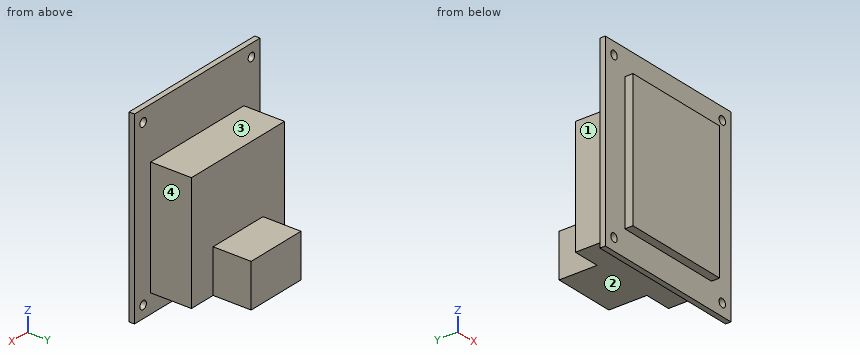
from build123d import *

# Parameters (mm, degrees)
SKETCH_1_W                  = 58
SKETCH_1_H                  = 69
EXTRUDE_351_DEPTH           = 2
SKETCH_2_W                  = 43
SKETCH_2_H                  = 43
EXTRUDE_607_DEPTH           = 15
SKETCH_3_W                  = 23
SKETCH_3_H                  = 16
EXTRUDE_850_DEPTH           = 14
SKETCH_4_W                  = 40
SKETCH_4_H                  = 50
EXTRUDE_1071_DEPTH          = 3
CUT_EXTRUDE_1381_DEPTH      = 54.593376456
CUT_EXTRUDE_1381_DEPTH_BACK = 54.593376456
SKETCH_7_R                  = 1.5


with BuildPart() as part:
    # Эскиз1 → Extrude 351 (new body)
    with BuildSketch(Plane.XZ):
        Rectangle(SKETCH_1_W, SKETCH_1_H)
    extrude(amount=-EXTRUDE_351_DEPTH)

    # Эскиз2 → Extrude 607 (add)
    with BuildSketch(Plane(origin=(0, 2, 0), x_dir=(-1, 0, 0), z_dir=(0, 1, 0))):
        with Locations((0, -6)):
            Rectangle(SKETCH_2_W, SKETCH_2_H)
    extrude(amount=EXTRUDE_607_DEPTH)

    # Эскиз3 → Extrude 850 (add)
    with BuildSketch(Plane(origin=(0, 17, 0), x_dir=(-1, 0, 0), z_dir=(0, 1, 0))):
        with Locations((0, -19.5)):
            Rectangle(SKETCH_3_W, SKETCH_3_H)
    extrude(amount=EXTRUDE_850_DEPTH)

    # Эскиз4 → Extrude 1071 (add)
    with BuildSketch(Plane.XZ):
        Rectangle(SKETCH_4_W, SKETCH_4_H)
    extrude(amount=EXTRUDE_1071_DEPTH)

    # Эскиз7 → Cut-Extrude 1381 (cut, two sides: drawn at the far end of the back side and taken through both)
    with BuildSketch(Plane(origin=(0, 2, 0), x_dir=(1, 0, 0), z_dir=(0, 1, 0)).offset(-CUT_EXTRUDE_1381_DEPTH_BACK)):
        with Locations(Location((-25, 30, 0), (0, 0, 90))):
            Circle(SKETCH_7_R)
        with Locations(Location((25, 30, 0), (0, 0, 90))):
            Circle(SKETCH_7_R)
        with Locations(Location((25, -30, 0), (0, 0, 90))):
            Circle(SKETCH_7_R)
        with Locations(Location((-25, -30, 0), (0, 0, 90))):
            Circle(SKETCH_7_R)
    extrude(amount=CUT_EXTRUDE_1381_DEPTH + CUT_EXTRUDE_1381_DEPTH_BACK, mode=Mode.SUBTRACT)


solid = part.part
Can you work these out from the model? Positions are in its coordinate system, mm. Face numbers are marked on the shaded views. A direction names the side the tool comes from. Round coordinates to 2 decimals unless told otherwise and drop trailing zeros. Loops run counter-clockwise (first coordinate to the right, second up) from the corner with the lowest first, then second, coordinate; pieces in that order, holes last. Notation, with made-up numbers: (78.25, -14) - (98.25, -14) arc R20 cw to (98.25, -5) - close; hole circle Ø4 at (6, -33). An arc over 180 degrees is marked (long way). Answer in a Markdown table with one row per item. Add a question column.
Q1. I want a section at B-B on z = -30. List the corners of the cut face in (x, y) for me.
Q2. I want a section at A-A on x = 25. List the corners of the cut face in (y, z) for me.
Q3. I want a section at D-D on x = 4. List the corners of the cut face in (y, z) for me, and give its area (3 significant figures).
Q4. I need wall thicknesses on L1, parallel to X at y = 0.9, z = -30; L2, parallel to Y at x = -12, z = 7.5; L3, parallel to X at y = 13, z = 2. Which ranges of each line are inside material? Lowest first, please.
Q5. Which directions (+Z, -Z, +X, -X, +Y, -Y) give clear straight access to the entire face, cutting with the end or side of a thin tool? Please do the marked faces 1, 2, 3 and 4.
Q6. For pin 1 Ø4.5 at (y, z) = (7.5, -6) entering from -X; pin 2 Ø11 at (x, y) = (2, 22) entering from +Z; pin 3 Ø1 at (x, y) = (-3.5, 17.5) entering from -Z, each with a flat end and sliding along its axis, tell me the tip position at first contact or that it passes through.
Q7. I want a section at C-C on z = -22. List the corners of the cut face in (x, y) for me.
A:
| question | item | result |
|---|---|---|
| 1 | outline | (-29, 0) - (-26.5, 0) - (-26.5, 2) - (-29, 2) - close; (-23.5, 0) - (23.5, 0) - (23.5, 2) - (-23.5, 2) - close; (26.5, 0) - (29, 0) - (29, 2) - (26.5, 2) - close |
| 2 | outline | (0, -34.5) - (2, -34.5) - (2, -31.5) - (0, -31.5) - close; (0, -28.5) - (2, -28.5) - (2, 28.5) - (0, 28.5) - close; (0, 31.5) - (2, 31.5) - (2, 34.5) - (0, 34.5) - close |
| 3 | outline | (-3, -25) - (0, -25) - (0, -34.5) - (2, -34.5) - (2, -27.5) - (31, -27.5) - (31, -11.5) - (17, -11.5) - (17, 15.5) - (2, 15.5) - (2, 34.5) - (0, 34.5) - (0, 25) - (-3, 25) - close |
| 3 | area | 1,160 mm^2 |
| 4 | L1 | -29 to -26.5, -23.5 to 23.5, 26.5 to 29 |
| 4 | L2 | -3 to 17 |
| 4 | L3 | -21.5 to 21.5 |
| 5 | face 1 | +Z, -Z, -X, +Y |
| 5 | face 2 | -Z, +X, -X, +Y |
| 5 | face 3 | +Z, +X, -X, +Y |
| 5 | face 4 | +Z, -Z, +X, +Y |
| 6 | pin 1 | x = -21.5 |
| 6 | pin 2 | z = 15.5 |
| 6 | pin 3 | z = -27.5 |
| 7 | outline | (-29, 0) - (-20, 0) - (-20, -3) - (20, -3) - (20, 0) - (29, 0) - (29, 2) - (21.5, 2) - (21.5, 17) - (11.5, 17) - (11.5, 31) - (-11.5, 31) - (-11.5, 17) - (-21.5, 17) - (-21.5, 2) - (-29, 2) - close |
